Verification items for the finished model (mm, model axes). A direction names the side the tool comes from. Give positions to 0.01 mm unless a question says otherwise; leave off trailing zeros. Write each loop counter-clockwise with the first axis right and the second up, starting at its lowest first coordinate (ties: lowest second). Pieces come first, ordered by that corner, then holes. Notation, with made-up numbers: M -16,20.25 L 16,20.25 A3 ccw 16,25.25 Z; hole C -14,1.5 d7. An arc over 180 degrees is marked long. Answer as a JSON object with one key per item and string values.
```python
from build123d import *

# Parameters (mm, degrees)
SKETCH1_R           = 15.875
SKETCH1_R_2         = 1.75
SKETCH1_W           = 25.4
SKETCH1_H           = 17.78
SKETCH1_R_3         = 1.27
BOSS_EXTRUDE1_DEPTH = 2.54
SKETCH2_R           = 3.175
SKETCH2_R_2         = 1.75
BOSS_EXTRUDE2_DEPTH = 5.974999988
SKETCH3_R           = 3
BOSS_EXTRUDE3_DEPTH = 17.61998


with BuildPart() as part:
    # Sketch1 → Boss-Extrude1 (new body)
    # profile 1 of 2: a face of its own
    with BuildSketch(Plane(origin=(0, 0, 0), x_dir=(1, 0, 0), z_dir=(0, 1, 0))):
        with Locations(Location((12.7, 8.89, 0), (0, 0, 270))):
            Circle(SKETCH1_R)
        with Locations(Location((12.7, 21.59, 0), (0, 0, 270))):
            Circle(SKETCH1_R_2, mode=Mode.SUBTRACT)
        with Locations(Location((12.7, -3.81, 0), (0, 0, 270))):
            Circle(SKETCH1_R_2, mode=Mode.SUBTRACT)
        with Locations((12.7, 8.89)):
            Rectangle(SKETCH1_W, SKETCH1_H, mode=Mode.SUBTRACT)
    # profile 2 of 2: a face of its own
    with BuildSketch(Plane(origin=(0, 0, 0), x_dir=(1, 0, 0), z_dir=(0, 1, 0))):
        with Locations((12.7, 8.89)):
            Rectangle(SKETCH1_W, SKETCH1_H)
        with Locations(Location((22.86, 15.24, 0), (0, 0, 270))):
            Circle(SKETCH1_R_3, mode=Mode.SUBTRACT)
        with Locations(Location((2.54, 15.24, 0), (0, 0, 270))):
            Circle(SKETCH1_R_3, mode=Mode.SUBTRACT)
        with Locations(Location((22.86, 2.54, 0), (0, 0, 270))):
            Circle(SKETCH1_R_3, mode=Mode.SUBTRACT)
        with Locations(Location((2.54, 2.54, 0), (0, 0, 270))):
            Circle(SKETCH1_R_3, mode=Mode.SUBTRACT)
    extrude(amount=BOSS_EXTRUDE1_DEPTH)

    # Sketch2 → Boss-Extrude2 (add)
    # profile 1 of 2: a face of its own
    with BuildSketch(Plane(origin=(0, 2.54, 0), x_dir=(1, 0, 0), z_dir=(0, 1, 0))):
        with Locations(Location((12.7, 21.59, 0), (0, 0, 89.999491582))):
            Circle(SKETCH2_R)
        with Locations(Location((12.7, 21.59, 0), (0, 0, 270))):
            Circle(SKETCH2_R_2, mode=Mode.SUBTRACT)
    # profile 2 of 2: a face of its own
    with BuildSketch(Plane(origin=(0, 2.54, 0), x_dir=(1, 0, 0), z_dir=(0, 1, 0))):
        with Locations(Location((12.7, -3.81, 0), (0, 0, 269.999491581))):
            Circle(SKETCH2_R)
        with Locations(Location((12.7, -3.81, 0), (0, 0, 270))):
            Circle(SKETCH2_R_2, mode=Mode.SUBTRACT)
    extrude(amount=BOSS_EXTRUDE2_DEPTH)

    # Sketch3 → Boss-Extrude3 (add)
    with BuildSketch(Plane.XZ):
        with Locations(Location((12.7, -8.89, 0), (0, 0, 90))):
            Circle(SKETCH3_R)
    extrude(amount=BOSS_EXTRUDE3_DEPTH)


solid = part.part
```
1) Thickness scan on L1, parallel to X at y = 1.85, z = -15.24; L2, parallel to Z at x = 14, y = 1.5; L3, parallel to Y at x = 21.5, z = 1.5. Record the ranges inside material, lowest first.
Completed:
{"L1": "x = -1.85 to 1.27, 3.81 to 21.59, 24.13 to 27.25", "L2": "z = -24.71 to -22.76, -20.42 to 2.64, 4.98 to 6.93", "L3": "y = 0 to 2.54"}
2) Section check D-D on y = -9. Record the boundary of the cut face in (x, z).
Completed:
{"outline": "C 12.7,-8.89 d6"}
3) Section check A-A on z = 3.81. Record the boundary of the cut face in (x, y) (3 decimals), and give its area (3 significant figures).
Completed:
{"outline": "M 3.175,0 L 10.95,0 L 10.95,8.515 L 9.525,8.515 L 9.525,2.54 L 3.175,2.54 Z; M 14.45,0 L 22.225,0 L 22.225,2.54 L 15.875,2.54 L 15.875,8.515 L 14.45,8.515 Z", "area": "56.5 mm2"}
4) Section check C-C on z = -9.5. Record the boundary of the cut face in (x, y), and give its area (3 significant figures).
Completed:
{"outline": "M -3.16,0 L 9.76,0 L 9.76,-17.62 L 15.64,-17.62 L 15.64,0 L 28.56,0 L 28.56,2.54 L -3.16,2.54 Z", "area": "184 mm2"}
5) Section check B-B on x = 3. Record the boundary of the cut face in (y, z).
Completed:
{"outline": "M 0,-21.46 L 2.54,-21.46 L 2.54,-16.42 L 0,-16.42 Z; M 0,-14.06 L 2.54,-14.06 L 2.54,-3.72 L 0,-3.72 Z; M 0,-1.36 L 2.54,-1.36 L 2.54,3.68 L 0,3.68 Z"}
6) Release check for a two-part mould opening along Z. For faces 1 (the face through (16, 0, -9)), 2 (the face through (17.47, 1.25, 6.25)), 3 (the face through (1.77, 1.25, -16.25)), 4 (the face through (1.3, 1.25, -2.82)) record: pulls with the +Z half, pulls with the -Z half, needs draft (parallel to the pull), parting line crosses it, or undercut.
Completed:
{"face 1": "needs draft", "face 2": "parting line crosses it", "face 3": "undercut", "face 4": "undercut"}
7) Go/stop test with flat-tipped pins: pin 1 (8 mm diameter, centred on x = 21.5, z = -8.5, fed in from +Y); pin 2 (1 mm diameter, centred on x = 6.5, z = -18.5, fed in from -Y); pin 3 (12 mm diameter, centred on y = -10.5, z = -14.5, fed in from +X). Record where each tip stops, or that it passes through.
Completed:
{"pin 1": "stops at y = 2.54", "pin 2": "stops at y = 0", "pin 3": "stops at x = 15.7"}
8) Access from +Z, -Z, +X, -X, +Y, -Y to the whole of each face (thin tool, end or side, straight path). Record for faces 5 (the face through (10.77, 5.49, 1.29)), 6 (the face through (23.718, 1.252, -16.176)), 7 (the face through (10.17, -8.69, -7.28)).
Completed:
{"face 5": "+Y", "face 6": "+Y, -Y", "face 7": "-Y"}
